The listing builds one solid part. Answer for the finished solid, in the listing's coordinates (mm). A direction names the side the tool comes from. Coordinates: 2 decimals unless noted, no trailing zeros. Loops run counter-clockwise (first coordinate to the right, second up) from the corner with the lowest first, then second, coordinate; pieces in that order, holes last. Notation, with made-up numbers: M 46.25,-11 L 95.25,-11 A20 ccw 95.25,25 Z; hole C 26.25,73.25 d5. An arc over 180 degrees is marked long. Answer as CSV lines item,"result". Start each with the question number.
Autodesk Inventor part; units mm, degrees
ref_plane "YZ Plane" through (0, 0, 0) normal (1, 0, 0) x (0, 1, 0)
ref_plane "XZ Plane" through (0, 0, 0) normal (0, 1, 0) x (-1, 0, 0)
ref_plane "XY Plane" through (0, 0, 0) normal (0, 0, 1) x (1, 0, 0)
sketch "Sketch1" plane through (0, 0, 0) normal (0, 1, 0) x (-1, 0, 0)
  circle A0 centre (0, 0) radius 4.3
  dimension "d0" = 8.6
extrude "Extrusion1" add sketch "Sketch1" along normal blind 8
sketch "Sketch2" plane through (0, 8, 0) normal (0, 1, 0) x (1, 0, 0)
  circle A0 centre (0, 0) radius 4.45
  dimension "d3" = 8.9
extrude "Extrusion2" add sketch "Sketch2" along normal blind 5
sketch "Sketch3" plane through (0, 13, 0) normal (0, 1, 0) x (1, 0, 0)
  line L0 (-3.4193, -0.0029) -> (1.6902, -2.9529)
  line L1 (1.6902, -2.9529) -> (1.6902, 2.9471)
  line L2 (1.6902, 2.9471) -> (-3.4193, -0.0029)
  point P0 (0, 0)
  dimension "d6" = 5.9
  dimension "d7" = 5.9
  dimension "d8" = 5.9
extrude "Extrusion3" add sketch "Sketch3" along normal blind 10
equation "\"d7\" = d6"
equation "\"d8\" = d6"
properties part number "TriangleAdapter"
Item 1: Section A-A on z = 3.25 is taken. Determine the outline of the cut face in (x, y).
Item 2: Section C-C on y = 6.75 is taken. Determine the outline of the cut face in (x, z).
Item 3: For faces 1 (the face through (4.296, 3.944, -0.189)), 2 (the face through (1.69, 18, 0)), 3 (the face through (-0.965, 10.465, -4.344)), 4 (the face through (-0.9, 17.93, 1.457)), 5 (the face through (-0.83, 17.93, -1.49)), determine the directions among +Z, -Z, +X, -X, +Y, -Y from which every point of the face is accessible in a straight line to the end or side of a thin tool.
Item 4: Section D-D on z = 2.25 is taken. Determine the outline of the cut face in (x, y).
Item 5: Section B-B on x = -1.75 is taken. Determine the outline of the cut face in (y, z), then the cut area to 3 significant figures.
Item 6: Consider line 1 (Y direction, x = -1.25, z = 2.5); line 2 (Z direction, x = -3, y = 13.75); line 3 (X direction, y = 5.5, z = -0.5). Determine where each line is inside the solid, lowest interval first.
Item 7: Each of these flat-tipped pins is pushed along its axis until it touches: P1, Ø4, axis at x = 2.5, z = 3, coming from the -Y side; P2, Ø1.5, axis at x = -2, y = 15.5, coming from the +Z side; P3, Ø1, axis at y = 2.5, z = -3, coming from the -X side; P4, Ø1.5, axis at y = 12.5, z = -2, coming from the -X side. Where does it stop, or does it pass through?
Results are:
1,outline,"M -3.04,8 L -2.82,8 L -2.82,0 L 2.82,0 L 2.82,8 L 3.04,8 L 3.04,13 L -3.04,13 Z"
2,outline,"C 0,0 d8.6"
3,face 1,"-Y"
3,face 2,"+Z, -Z, +X, +Y"
3,face 3,"+Y, -Y"
3,face 4,"+Z, -X, +Y"
3,face 5,"-Z, -X, +Y"
4,outline,"M -3.84,8 L -3.66,8 L -3.66,0 L 3.66,0 L 3.66,8 L 3.84,8 L 3.84,13 L 1.69,13 L 1.69,23 L 0.47,23 L 0.47,13 L -3.84,13 Z"
5,outline,"M 0,-3.93 L 8,-3.93 L 8,-4.09 L 13,-4.09 L 13,-0.96 L 23,-0.96 L 23,0.97 L 13,0.97 L 13,4.09 L 8,4.09 L 8,3.93 L 0,3.93 Z"
5,area,"123 mm²"
6,line 1,"0 to 13"
6,line 2,"-0.24 to 0.24"
6,line 3,"-4.27 to 4.27"
7,P1,"y = 0"
7,P2,"z = 1.26"
7,P3,"x = -3.5"
7,P4,"x = -4.27"
